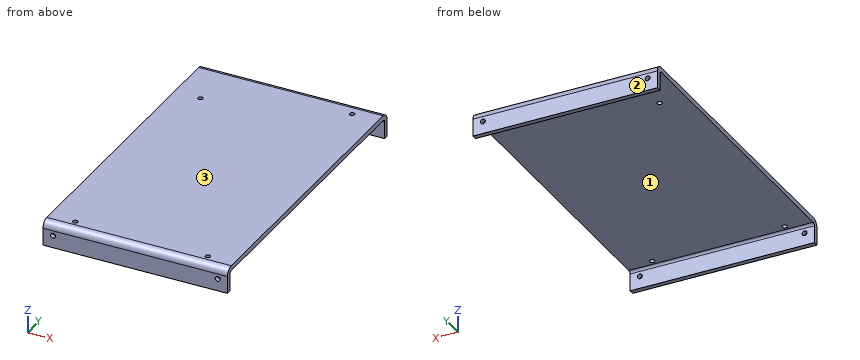
from build123d import *

# Parameters (mm, degrees)
SKETCH1_W                      = 125
SKETCH1_H                      = 74.5
SKETCH1_R                      = 1
BASE_FLANGE1_DEPTH             = 2
EDGE_FLANGE2_STRIP_W           = 9.9304
EDGE_FLANGE2_STRIP_H           = 2
EDGE_FLANGE2_STRIP_CUT_DEPTH   = 74.5
EDGE_FLANGE2_STRIP_2_W         = 9.9304
EDGE_FLANGE2_STRIP_2_H         = 2
EDGE_FLANGE2_STRIP_CUT_2_DEPTH = 74.5
EDGE_FLANGE2_DEPTH             = 74.5
EDGE_FLANGE2_BEND_DEPTH        = 74.5
SKETCH20_R                     = 1
CUT_EXTRUDE2_DEPTH             = 141.78707327


# Sheet-metal steps are written as plain solids
with BuildPart() as part:
    # Sketch1 → Base-Flange1 (new body)
    with BuildSketch(Plane(origin=(0, 0, 0), x_dir=(0, 1, 0), z_dir=(0, 0, 1))):
        with Locations((-55.5, 26.75)):
            Rectangle(SKETCH1_W, SKETCH1_H)
        with Locations(Location((0, 0, 0), (0, 0, 270))):
            Circle(SKETCH1_R, mode=Mode.SUBTRACT)
        with Locations(Location((-113, 0, 0), (0, 0, 270))):
            Circle(SKETCH1_R, mode=Mode.SUBTRACT)
        with Locations(Location((-113, 53.5, 0), (0, 0, 270))):
            Circle(SKETCH1_R, mode=Mode.SUBTRACT)
        with Locations(Location((-15, 53.5, 0), (0, 0, 270))):
            Circle(SKETCH1_R, mode=Mode.SUBTRACT)
    extrude(amount=-BASE_FLANGE1_DEPTH)

    # Edge-Flange2 strip (across the edge) → Edge-Flange2 strip cut (cut)
    with BuildSketch(Plane(origin=(10.5, -118, -2), x_dir=(0, 1, 0), z_dir=(-1, 0, 0))):
        with Locations((-2, -1)):
            Rectangle(EDGE_FLANGE2_STRIP_W, EDGE_FLANGE2_STRIP_H)
    extrude(amount=EDGE_FLANGE2_STRIP_CUT_DEPTH, mode=Mode.SUBTRACT)

    # Edge-Flange2 strip 2 (across the edge) → Edge-Flange2 strip cut 2 (cut)
    with BuildSketch(Plane(origin=(-64, 7, -2), x_dir=(0, -1, 0), z_dir=(1, 0, 0))):
        with Locations((-2, -1)):
            Rectangle(EDGE_FLANGE2_STRIP_2_W, EDGE_FLANGE2_STRIP_2_H)
    extrude(amount=EDGE_FLANGE2_STRIP_CUT_2_DEPTH, mode=Mode.SUBTRACT)

    # Edge-Flange2 section (across the edge) → Edge-Flange2 (add)
    with BuildSketch(Plane(origin=(10.5, -118, -2), x_dir=(0, 1, 0), z_dir=(-1, 0, 0))):
        with BuildLine():
            Line((0, 0.9652), (0, 8))
            Line((0, 8), (2, 8))
            Line((2, 8), (2, 0.9652))
            ThreePointArc((2, 0.9652), (2.282700535, 0.282700535), (2.9652, 0))
            Line((2.9652, 0), (2.9652, -2))
            ThreePointArc((2.9652, -2), (0.868486972, -1.131513028), (0, 0.9652))
        make_face()
    extrude(amount=EDGE_FLANGE2_DEPTH)

    # Edge-Flange2 section 2 (across the edge) → Edge-Flange2 bend (add)
    with BuildSketch(Plane(origin=(-64, 7, -2), x_dir=(0, -1, 0), z_dir=(1, 0, 0))):
        with BuildLine():
            Line((0, 0.9652), (0, 8))
            Line((0, 8), (2, 8))
            Line((2, 8), (2, 0.9652))
            ThreePointArc((2, 0.9652), (2.282700535, 0.282700535), (2.9652, 0))
            Line((2.9652, 0), (2.9652, -2))
            ThreePointArc((2.9652, -2), (0.868486972, -1.131513028), (0, 0.9652))
        make_face()
    extrude(amount=EDGE_FLANGE2_BEND_DEPTH)

    # Sketch20 → Cut-Extrude2 (cut, through all)
    with BuildSketch(Plane.XZ.offset(118)):
        with Locations(Location((-60, -5, 0), (0, 0, 270))):
            Circle(SKETCH20_R)
        with Locations(Location((6.5, -5, 0), (0, 0, 270))):
            Circle(SKETCH20_R)
    extrude(amount=-CUT_EXTRUDE2_DEPTH, mode=Mode.SUBTRACT)


solid = part.part
Can you work these out from the model? Positions are in its coordinate system, mm. Face numbers are marked on the shaded views. Give positions to 0.01 mm unless a question says otherwise; leave off trailing zeros. Order: outer loops, then holes, each group sorted by start corner. A loop starts at its lowest first (then second) coordinate and runs counter-clockwise, first axis right, second up. Notation, with made-up numbers: M -36.5,-21.75 L -17.5,-21.75 A17 ccw -17.5,-0.75 Z; hole C 51.5,-38 d8. An arc over 180 degrees is marked long. Use one line per item in the form item = value. Start each with the question number.
Item 1: If we section it at A-A (x = -42): Write out the boundary of the cut face in (y, z), then the cut area to 3 significant figures.
Item 2: If we section it at B-B (y = -61): Write out the boundary of the cut face in (x, z), then the cut area to 3 significant figures.
Item 3: If I drill on line 1 along X through (y, z) = (5.65, -5); line 2 along Y through (x, z) = (-39, -2.75); line 3 along Z through (x, y) = (-57, -52.5), over which ranges is the centre line in solid material (lowest first)?
Item 4: Will these pins go through, and if not, where does the flat tip stop? pin 1 Ø4 at (x, z) = (-48.5, -2) entering from -Y; pin 2 Ø2.5 at (x, y) = (0, 0) entering from -Z.
Item 5: We'd pull the mould along Y, two halves only. Please class the marked faces 1, 2 and 3: +Y half, -Y half, draft (parallel to the pull), parting line (faces both ways), or undercut.
Outcome:
q1.outline = M -118,-10 L -116,-10 L -116,-2.97 A0.97 cw -115.03,-2 L 4.03,-2 A0.97 cw 5,-2.97 L 5,-10 L 7,-10 L 7,-2.97 A2.97 ccw 4.03,0 L -115.03,0 A2.97 ccw -118,-2.97 Z
q1.area = 279 mm2
q2.outline = M -64,-2 L 10.5,-2 L 10.5,0 L -64,0 Z
q2.area = 149 mm2
q3.line_1 = -64 to -61, -59 to 5.5, 7.5 to 10.5
q3.line_2 = -117.99 to -115.98, 4.98 to 6.99
q3.line_3 = -2 to 0
q4.pin_1 = -118
q4.pin_2 = -2
q5.face_1 = undercut
q5.face_2 = +Y half
q5.face_3 = draft
